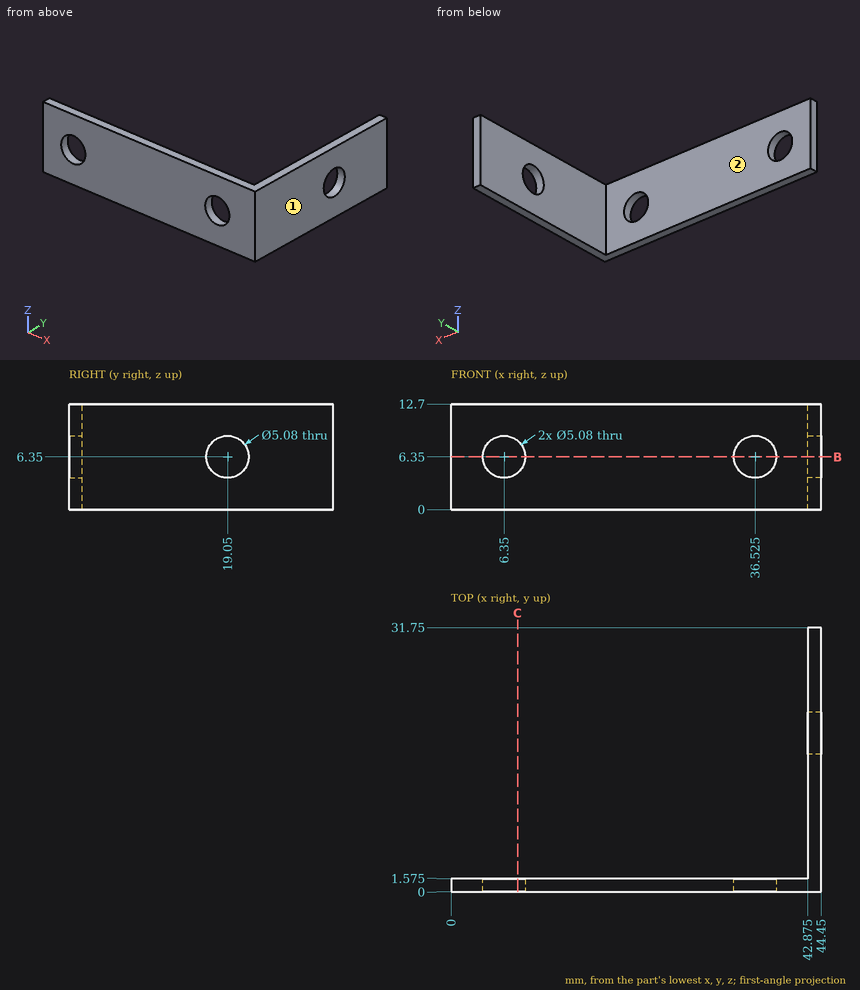
Verification items for this drawing (mm, ordinates from the low corner). A direction names the side the tool comes from. Round coordinates to 2 decimals unless told otherwise and drop trailing zeros. Loops run counter-clockwise (first coordinate to the right, second up) from the corner with the lowest first, then second, coordinate; pieces in that order, holes last. Notation, with made-up numbers: (17.25, -38.75) -> (26.25, -38.75) arc R17 ccw to (26.25, -16.75) -> close; hole circle Ø3 at (-18.5, 64). An arc over 180 degrees is marked (long way). Write item = value, one per line. Start each with the question number.
1) Sectioned sample at B-B, the plane z = 6.35. State how many separate pieces and enclosed holes the cut face has.
2) Thickness scan on probe 1 along Y at (x, z) = (44.05, 6.35); probe 2 along Z at (x, y) = (43, 19); probe 3 along Y at (x, z) = (37, 11.75) (1 decimal). Record the ranges inside material, lowest first.
3) Sectioned sample at C-C, the plane x = 8. Record the cut outline in (y, z) (1 decimal), plus the area to 3 significant figures.
4) Gauge pin test, flat end, axial feed: pin 1 Ø4 at (y, z) = (13.5, 9) entering from -X (3 decimals). Record the tip position at first contact, or that the pin passes through.
5) Set-up check for the marked faces 1 and 2: record each of +Z, -Z, +X, -X, +Y, -Y from which the full face is reachable in a straight line by a thin tool's end or side.
Results are:
q1.separate_pieces = 4
q1.enclosed_holes = 0
q2.probe_1 = 0 to 16.51, 21.59 to 31.75
q2.probe_2 = 0 to 3.81, 8.89 to 12.7
q2.probe_3 = 0 to 1.6
q3.outline = (0, 0) -> (1.6, 0) -> (1.6, 4.4) -> (0, 4.4) -> close; (0, 8.3) -> (1.6, 8.3) -> (1.6, 12.7) -> (0, 12.7) -> close
q3.area = 13.9 mm^2
q4.pin_1 = 42.875
q5.face_1 = +Z, -Z, +X, +Y, -Y
q5.face_2 = +Z, -Z, -X, +Y
